Job drawing, mm, ordinate dimensions from the low corner. One solid piece. A direction names the side the tool comes from. Round coordinates to 2 decimals unless told otherwise and drop trailing zeros. Loops run counter-clockwise (first coordinate to the right, second up) from the corner with the lowest first, then second, coordinate; pieces in that order, holes last. Notation, with made-up numbers: M -13,43.5 L 22,43.5 A10 ccw 22,57.5 Z; hole C 66.25,61 d9. An arc over 180 degrees is marked long. Use one line per item in the form item = value.
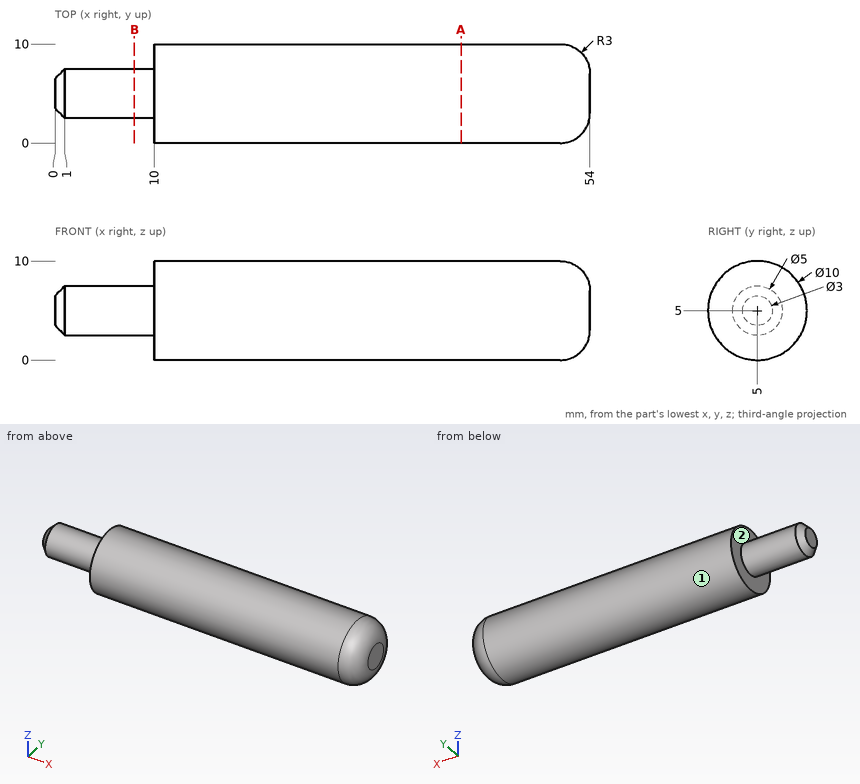
1. Drop flat-ended pins along their axis: P1, Ø3, axis at x = 36.5, z = 7.5, coming from the -Y side; P2, Ø3, axis at y = 8, z = 3.5, coming from the -X side; P3, Ø1.5, axis at x = 5.5, z = 6, coming from the -Y side. Give the stop position or say it passes through.
Completed:
P1 = 0.1
P2 = 0.35
P3 = 2.51
2. Probe line 1 along Y through (x, z) = (12.5, 4.75); line 2 along Y through (x, z) = (4.5, 3.5); line 3 along X through (y, z) = (9, 5.5). List the from-to ranges inside material, lowest first. Write a range as from..to.
Completed:
line_1 = 0.01..9.99
line_2 = 3..7
line_3 = 10..53.21
3. Cut at B-B on x = 8. Write the cut outline in (y, z), and give its area (3 significant figures).
Completed:
outline = C 5,5 d5
area = 19.6 mm2
4. Tool access for the marked faces 1 and 2: list every direction of +Z, -Z, +X, -X, +Y, -Y with a clear straight run to the whole face (end or side of a thin tool).
Completed:
face_1 = +X, -X
face_2 = -X
5. Cut at A-A on x = 41. Write the cut outline in (y, z).
Completed:
outline = C 5,5 d10
